```python
from build123d import *

# Parameters (mm, degrees)
F0_R     = 6.75
F0_R_2   = 6.375
F1_DEPTH = 100
F2_R     = 6.75
F3_DEPTH = 1
F4_R     = 6.75
F5_DEPTH = 1


with BuildPart() as f1:
    # F0 (on Right) → F1 (new body)
    with BuildSketch(Plane.YZ):
        Circle(F0_R)
        Circle(F0_R_2, mode=Mode.SUBTRACT)
    extrude(amount=F1_DEPTH)

    # F2 (on face) → F3 (join)
    with BuildSketch(Plane(origin=(0, 0, 0), x_dir=(0, -1, 0), z_dir=(-1, 0, 0))):
        Circle(F2_R)
    extrude(amount=F3_DEPTH)

    # F4 (on face) → F5 (join)
    with BuildSketch(Plane.YZ.offset(100)):
        Circle(F4_R)
    extrude(amount=F5_DEPTH)


solid = f1.part
```
Input: part model. Units: mm. Frame: model coordinates. Round coordinates to 2 decimals unless told otherwise and drop trailing zeros. Order: outer loops, then holes, each group sorted by start corner. A loop starts at its lowest first (then second) coordinate and runs counter-clockwise, first axis right, second up. Notation, with made-up numbers: (-7.75, -37.5) - (2.25, -37.5) arc R15 cw to (2.25, -31.5) - close; hole circle Ø1 at (-6.5, 67.25). An arc over 180 degrees is marked (long way). One line per question, with ' | ' between items. Start each with the question number.
1) Contact query for flat-ended pins moving along their axis: P1, Ø1, axis at x = 11, y = -3, coming from the +Z side; P2, Ø1, axis at x = 88.5, z = -1, coming from the -Y side. Output: stop coordinate, or through.
2) Ray query, probe 1 along Z at (x, y) = (40.5, 0) (3 decimals); probe 2 along X at (y, z) = (5.5, -0.5); probe 3 along Y at (x, z) = (26, 3.75). Return the intervals inside material, ascending.
3) Pull-direction query (X, two-part tool) for faces 1 (the flat face through (-1, 0, 0)), 2 (the flat face through (100, 0, 0)), 3 (the flat face through (101, 0, 0)); classes: +X half, -X half, draft (parallel to the pull), parting line (faces both ways), or undercut.
4) Cut plane C-C, the plane x = 6. Return the cut outline in (y, z) (3 decimals), then the cut area to 3 significant figures.
5) Cut plane A-A, the plane y = 0. Return the cut outline in (x, z) (3 decimals).
Worked out:
1) P1: stops at z = 6.27 | P2: stops at y = -6.73
2) probe 1: z = -6.75 to -6.375, 6.375 to 6.75 | probe 2: x = -1 to 0, 100 to 101 | probe 3: y = -5.61 to -5.16, 5.16 to 5.61
3) face 1: -X half | face 2: undercut | face 3: +X half
4) outline: circle Ø13.5 at (0, 0); hole circle Ø12.75 at (0, 0) | area: 15.5 mm^2
5) outline: (-1, -6.75) - (101, -6.75) - (101, 6.75) - (-1, 6.75) - close; hole (0, -6.375) - (100, -6.375) - (100, 6.375) - (0, 6.375) - close
